from build123d import *

# Parameters (mm, degrees)
SKETCH1_R               = 25
BOSS_EXTRUDE1_DEPTH     = 45
CUT_EXTRUDE1_START      = -40
CUT_EXTRUDE1_DEPTH      = 40
SKETCH3_R               = 5
BOSS_EXTRUDE2_DEPTH     = 2
CUT_EXTRUDE2_DEPTH      = 69.373971656
CUT_EXTRUDE2_DEPTH_BACK = 69.373971656
SKETCH4_R               = 5


with BuildPart() as part:
    # Sketch1 → Boss-Extrude1 (new body)
    with BuildSketch(Plane.XY):
        with Locations(Location((0, 0, 0), (0, 0, 180))):
            Circle(SKETCH1_R)
    extrude(amount=BOSS_EXTRUDE1_DEPTH)

    # Sketch2 → Cut-Extrude1 (cut)
    with BuildSketch(Plane.XY.offset(45).offset(CUT_EXTRUDE1_START)):
        with BuildLine():
            Line((-20, 15), (-20, -15))
            ThreePointArc((-20, -15), (0, -25), (20, -15))
            Line((20, -15), (20, 15))
            ThreePointArc((20, 15), (0, 25), (-20, 15))
        make_face()
    extrude(amount=CUT_EXTRUDE1_DEPTH, mode=Mode.SUBTRACT)

    # Sketch3 → Boss-Extrude2 (add)
    with BuildSketch(Plane(origin=(0, 0, 0), x_dir=(-1, 0, 0), z_dir=(0, 0, -1))):
        with Locations(Location((6.33, 7.66, 0), (0, 0, 180))):
            Circle(SKETCH3_R)
        with Locations(Location((-6.33, -7.66, 0), (0, 0, 180))):
            Circle(SKETCH3_R)
    extrude(amount=BOSS_EXTRUDE2_DEPTH)

    # Sketch4 → Cut-Extrude2 (cut, two sides: drawn at the far end of the back side and taken through both)
    with BuildSketch(Plane(origin=(-20, 0, 0), x_dir=(0, 0, -1), z_dir=(1, 0, 0)).offset(-CUT_EXTRUDE2_DEPTH_BACK)):
        with Locations((-33, 0)):
            Circle(SKETCH4_R)
    extrude(amount=CUT_EXTRUDE2_DEPTH + CUT_EXTRUDE2_DEPTH_BACK, mode=Mode.SUBTRACT)


solid = part.part
Work out the finished part from the listing and answer in its coordinate system (mm). A direction names the side the tool comes from. Give positions to 0.01 mm unless a question says otherwise; leave off trailing zeros. Loops run counter-clockwise (first coordinate to the right, second up) from the corner with the lowest first, then second, coordinate; pieces in that order, holes last. Notation, with made-up numbers: (-23.75, 26.25) -> (23.25, 26.25) arc R25 cw to (23.25, 57.25) -> close; hole circle Ø3 at (19.5, 73). An arc over 180 degrees is marked (long way). Use a Markdown table: item, result. Add a question column.
1. For faces 4 (the cylindrical face through (-10.3, 10.7, -1)), 5 (the flat face through (20, 0, 25)), 6 (the flat face through (22, 0, 45)), determine the directions among +Z, -Z, +X, -X, +Y, -Y from which every point of the face is accessible in a straight line to the end or side of a thin tool.
2. Section A-A on z = 34 is taken. Determine the outline of the cut face in (x, y).
3. Section D-D on x = 6.33 is taken. Determine the outline of the cut face in (y, z).
4. Flat-ended cylindrical pins translate along their axes: pin 1 Ø6 at (x, y) = (6.5, 19.5) entering from -Z; pin 2 Ø12 at (x, y) = (6.5, 4) entering from +Z; pin 3 Ø4 at (y, z) = (-16, 14) entering from -X. Find the tip coordinate at first contact, or state that the pin passes through.
5. Section B-B on y = 0 is taken. Determine the outline of the cut face in (x, z).
6. Section C-C on z = 16.5 is taken. Determine the outline of the cut face in (x, y), and give its area (3 significant figures).
7. Determine the mould class of faces 1 (the cylindrical face through (-23, 0, 38)), 2 (the cylindrical face through (8.637, -3.224, -0.986)), 3 (the flat face through (-22, 0, 45)) for opening direction Y: released by +Y, released by -Y, zero draft, split by the parting line, or undercut.
8. Find the intervals of material crossed by probe 1 along Z at (x, y) = (-23, 0); probe 2 along Z at (x, y) = (-8, -7.5); probe 3 along X at (y, z) = (-1.5, 6.5), in increasing order.
Results below:
| question | item | result |
|---|---|---|
| 1 | face 4 | -Z |
| 1 | face 5 | +Z, +Y, -Y |
| 1 | face 6 | +Z, +X, -X, +Y, -Y |
| 2 | outline | (-24.52, -4.9) arc R25 ccw to (-20, -15) -> (-20, -4.9) -> close; (-24.52, 4.9) -> (-20, 4.9) -> (-20, 15) arc R25 ccw to start; (20, -15) arc R25 ccw to (24.52, -4.9) -> (20, -4.9) -> close; (20, 4.9) -> (24.52, 4.9) arc R25 ccw to (20, 15) -> close |
| 3 | outline | (-24.19, 0) -> (-12.66, 0) -> (-12.66, -2) -> (-2.66, -2) -> (-2.66, 0) -> (24.19, 0) -> (24.19, 5) -> (-24.19, 5) -> close |
| 4 | pin 1 | stops at z = 0 |
| 4 | pin 2 | stops at z = 5 |
| 4 | pin 3 | stops at x = -20.71 |
| 5 | outline | (-25, 0) -> (25, 0) -> (25, 28) -> (20, 28) -> (20, 5) -> (-20, 5) -> (-20, 28) -> (-25, 28) -> close; (-25, 38) -> (-20, 38) -> (-20, 45) -> (-25, 45) -> close; (20, 38) -> (25, 38) -> (25, 45) -> (20, 45) -> close |
| 6 | outline | (-20, -15) -> (-20, 15) arc R25 ccw to start; (20, -15) arc R25 ccw to (20, 15) -> close |
| 6 | area | 204 mm^2 |
| 7 | face 1 | undercut |
| 7 | face 2 | split by the parting line |
| 7 | face 3 | zero draft |
| 8 | probe 1 | z = 0 to 28, 38 to 45 |
| 8 | probe 2 | z = 0 to 5 |
| 8 | probe 3 | x = -24.95 to -20, 20 to 24.95 |
